Print and shaded views of the part. All mm, measured from the part's lowest x, y and z. A direction names the side the tool comes from. Round coordinates to 2 decimals unless told otherwise and drop trailing zeros. Loops run counter-clockwise (first coordinate to the right, second up) from the corner with the lowest first, then second, coordinate; pieces in that order, holes last. Notation, with made-up numbers: (23, 2.25) - (58, 2.25) arc R10 ccw to (58, 6.25) - close; hole circle Ø5 at (-11.75, 68.25). An arc over 180 degrees is marked (long way). Answer as a JSON object with one key per item and string values.
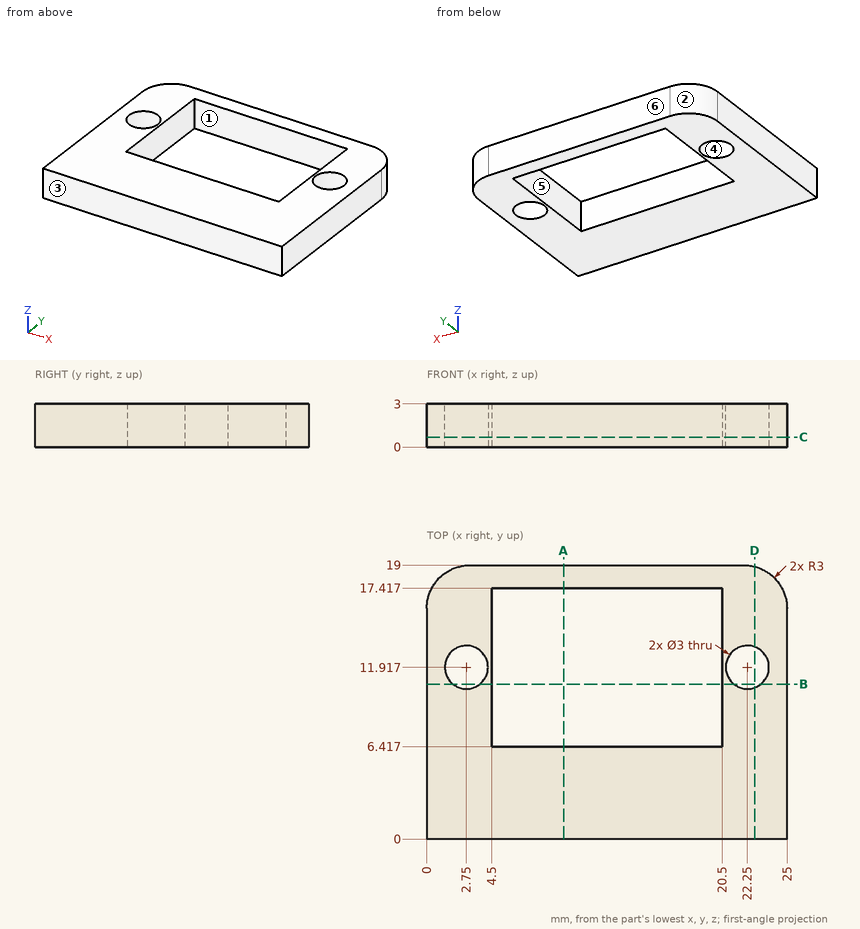
1) Slice it at A-A on x = 9.5. List the corners of the cut face in (y, z).
Values follow:
{"outline": "(0, 0) - (6.42, 0) - (6.42, 3) - (0, 3) - close; (17.42, 0) - (19, 0) - (19, 3) - (17.42, 3) - close"}
2) Slice it at D-D on x = 22.75. List the corners of the cut face in (y, z) (1 decimal).
Values follow:
{"outline": "(0, 0) - (10.5, 0) - (10.5, 3) - (0, 3) - close; (13.3, 0) - (18.9, 0) - (18.9, 3) - (13.3, 3) - close"}
3) Tool access for the marked faces 5 and 6: list every direction of +Z, -Z, +X, -X, +Y, -Y with a clear straight run to the whole face (end or side of a thin tool).
Values follow:
{"face 5": "+Z, -Z", "face 6": "+Z, -Z, +X, -X, +Y"}
4) Two-plate mould, pull along Y, no slides. Class the marked faces 1, 2, 3 and 4: pulls with the +Y half, pulls with the -Y half, needs draft (parallel to the pull), parting line crosses it, or undercut.
Values follow:
{"face 1": "undercut", "face 2": "pulls with the +Y half", "face 3": "pulls with the -Y half", "face 4": "undercut"}
5) Probe probe 1 along X at (y, z) = (12, 2.5); probe 2 along X at (y, z) = (8, 2.55); probe 3 along Y at (x, z) = (15, 0.6). List the from-to ranges inside material, lowest first.
Values follow:
{"probe 1": "0 to 1.25, 4.25 to 4.5, 20.5 to 20.75, 23.75 to 25", "probe 2": "0 to 4.5, 20.5 to 25", "probe 3": "0 to 6.42, 17.42 to 19"}
6) Slice it at C-C on z = 0.7. List the corners of the cut face in (x, y).
Values follow:
{"outline": "(0, 0) - (25, 0) - (25, 16) arc R3 ccw to (22, 19) - (3, 19) arc R3 ccw to (0, 16) - close; hole circle Ø3 at (2.75, 11.92); hole (4.5, 6.42) - (20.5, 6.42) - (20.5, 17.42) - (4.5, 17.42) - close; hole circle Ø3 at (22.25, 11.92)"}
7) Slice it at B-B on y = 10.75. List the corners of the cut face in (x, z).
Values follow:
{"outline": "(0, 0) - (1.81, 0) - (1.81, 3) - (0, 3) - close; (3.69, 0) - (4.5, 0) - (4.5, 3) - (3.69, 3) - close; (20.5, 0) - (21.31, 0) - (21.31, 3) - (20.5, 3) - close; (23.19, 0) - (25, 0) - (25, 3) - (23.19, 3) - close"}
